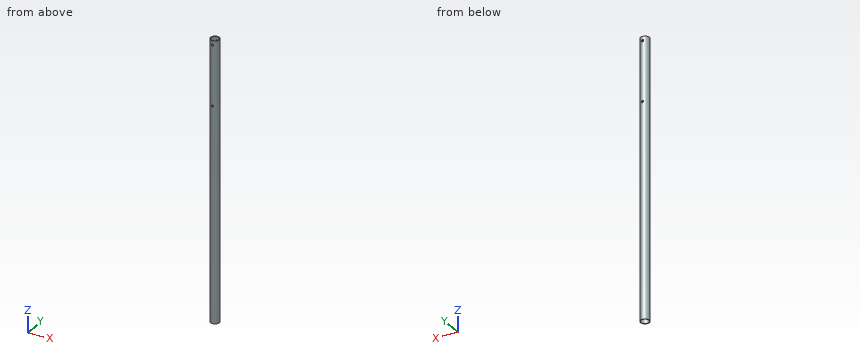
```python
from build123d import *

# Parameters (mm, degrees)
F0_R     = 12.7
F0_R_2   = 11.2
F1_DEPTH = 825.5
F2_R     = 3.175
F3_DEPTH = 12.7


with BuildPart() as f1:
    # F0 (on Top) → F1 (new body)
    with BuildSketch(Plane.XY):
        Circle(F0_R)
        Circle(F0_R_2, mode=Mode.SUBTRACT)
    extrude(amount=F1_DEPTH)

    # F2 (on Front) → F3 (cut, symmetric)
    with BuildSketch(Plane.XZ):
        with Locations((0, 812.8)):
            Circle(F2_R)
        with Locations((0, 635)):
            Circle(F2_R)
    extrude(amount=F3_DEPTH, both=True, mode=Mode.SUBTRACT)


solid = f1.part
```
Could you check a few things on this model? Use its own coordinates, in mm. Round coordinates to 2 decimals unless told otherwise and drop trailing zeros. Loops run counter-clockwise (first coordinate to the right, second up) from the corner with the lowest first, then second, coordinate; pieces in that order, holes last. Notation, with made-up numbers: M 85,-5 L 124,-5 A24 ccw 124,16 Z; hole C 12.5,38.25 d8. An arc over 180 degrees is marked long. Put each result on its own line as item: value.
Q1. I need wall thicknesses on probe 1 along Z at (x, y) = (0, 11.75) (3 decimals); probe 2 along Y at (x, z) = (1, 607.5); probe 3 along Y at (x, z) = (-5.5, 547). Which ranges of each line are inside material? Lowest first, please.
Check result:
probe 1: 0 to 631.825, 638.175 to 809.625, 815.975 to 825.5
probe 2: -12.66 to -11.16, 11.16 to 12.66
probe 3: -11.45 to -9.76, 9.76 to 11.45
Q2. For pin 1 (6 mm diameter, centred on x = -9.5, z = 470.5, fed in from -Y); pin 2 (2 mm diameter, centred on y = 8, z = 299.5, fed in from +X); pin 3 (5 mm diameter, centred on x = -8.5, z = 271, fed in from -Y), each with a flat end and sliding along its axis, tell me the tip position at first contact or that it passes through.
Check result:
pin 1: y = -10.91
pin 2: x = 10.6
pin 3: y = -11.19
Q3. Imagine slicing it at B-B (z = 263). Write out the boundary of the cut face in (x, y).
Check result:
outline: C 0,0 d25.4; hole C 0,0 d22.4
Q4. Imagine slicing it at A-A (y = 0). Write out the boundary of the cut face in (x, z), then the cut area to 3 significant figures.
Check result:
outline: M -12.7,0 L -11.2,0 L -11.2,825.5 L -12.7,825.5 Z; M 11.2,0 L 12.7,0 L 12.7,825.5 L 11.2,825.5 Z
area: 2,480 mm2
